from build123d import *

# Parameters (mm, degrees)
F1_DEPTH = 0.635


with BuildPart() as f1:
    # F0 (on Top) → F1 (new body)
    with BuildSketch(Plane.XY):
        with BuildLine():
            Line((-29.810913, 1.540789), (-31.016748, 0))
            Line((-31.016748, 0), (19.896272, 0))
            Line((19.896272, 0), (18.82442, 2.880605))
            Line((18.82442, 2.880605), (17.860188, 5.716184))
            Line((17.860188, 5.716184), (14.670988, 8.373851))
            Line((14.670988, 8.373851), (13.588352, 10.739779))
            ThreePointArc((13.588352, 10.739779), (14.154572, 11.638903), (13.104023, 11.798203))
            Line((13.104023, 11.798203), (12.573407, 12.957779))
            Line((12.573407, 12.957779), (9.713667, 15.340896))
            Line((9.713667, 15.340896), (6.230144, 13.197191))
            Line((6.230144, 13.197191), (3.148568, 11.455429))
            Line((3.148568, 11.455429), (1.540788, 12.795246))
            Line((1.540788, 12.795246), (0.818556, 12.795246))
            ThreePointArc((0.818556, 12.795246), (-4.276831, 15.082857), (-8.518913, 11.449555))
            Line((-8.518913, 11.449555), (-8.641816, 11.589411))
            Line((-8.641816, 11.589411), (-11.991355, 16.680711))
            Line((-11.991355, 16.680711), (-14.938951, 18.288492))
            Line((-14.938951, 18.288492), (-20.432198, 14.269044))
            Line((-20.432198, 14.269044), (-21.582795, 11.795261))
            ThreePointArc((-21.582795, 11.795261), (-22.634312, 11.642479), (-22.073679, 10.739861))
            Line((-22.073679, 10.739861), (-23.11183, 8.507834))
            Line((-23.11183, 8.507834), (-26.059426, 6.364127))
            Line((-26.059426, 6.364127), (-27.265261, 3.148568))
            Line((-27.265261, 3.148568), (-29.810913, 1.540789))
        make_face()
        Polygon((-25.742841, 6.123265), (-22.807967, 8.25772), (-20.128087, 14.019463), (-14.909113, 17.838224), (-12.257344, 16.391804), (-8.96011, 11.380007), (-8.92801, 11.337907), (-5.075081, 6.95354), (-3.355364, 3.514106), (-3.309465, 3.443231), (-0.804003, 0.381), (-30.234767, 0.381), (-29.551596, 1.253941), (-26.9535, 2.894843), align=None, mode=Mode.SUBTRACT)
        with BuildLine():
            Line((-3.717773, 5.090865), (-4.756348, 7.168017))
            Line((-4.756348, 7.168017), (-6.445825, 9.090525))
            Line((-6.445825, 9.090525), (-3.479574, 11.133942))
            Line((-3.479574, 11.133942), (-1.303058, 12.414246))
            Line((-1.303058, 12.414246), (1.402847, 12.414246))
            Line((1.402847, 12.414246), (2.869082, 11.192383))
            Line((2.869082, 11.192383), (-0.923488, 8.639836))
            Line((-0.923488, 8.639836), (-3.616762, 5.088058))
            ThreePointArc((-3.616762, 5.088058), (-3.667275, 5.089198), (-3.717773, 5.090865))
        make_face(mode=Mode.SUBTRACT)
        Polygon((-0.311727, 0.381), (-3.014587, 3.684495), (-3.506604, 4.668528), (-3.313175, 4.85785), (-0.658187, 8.359138), (3.081815, 10.876305), (3.130206, 10.914939), (3.336041, 11.123745), (6.423789, 12.868994), (9.680128, 14.872894), (12.262983, 12.720515), (14.324537, 8.215317), (14.427077, 8.081159), (17.533967, 5.492083), (18.463705, 2.757945), (18.467338, 2.747738), (19.347984, 0.381), align=None, mode=Mode.SUBTRACT)
        with BuildLine():
            ThreePointArc((-21.770268, 11.392193), (-21.766019, 11.363603), (-21.764598, 11.334734))
            ThreePointArc((-21.764598, 11.334734), (-22.351069, 11.305865), (-21.770268, 11.392193))
        make_face(mode=Mode.SUBTRACT)
        with BuildLine():
            Line((-3.684495, 11.455429), (-6.699082, 9.378714))
            Line((-6.699082, 9.378714), (-8.218903, 11.108165))
            ThreePointArc((-8.218903, 11.108165), (-4.466352, 14.664212), (0.353822, 12.795246))
            Line((0.353822, 12.795246), (-1.406807, 12.795246))
            Line((-1.406807, 12.795246), (-3.684495, 11.455429))
        make_face(mode=Mode.SUBTRACT)
        with BuildLine():
            ThreePointArc((13.831154, 11.37468), (13.631239, 11.126505), (13.346187, 11.268991))
            ThreePointArc((13.346187, 11.268991), (13.523069, 11.622855), (13.831154, 11.37468))
        make_face(mode=Mode.SUBTRACT)
    extrude(amount=F1_DEPTH)


solid = f1.part
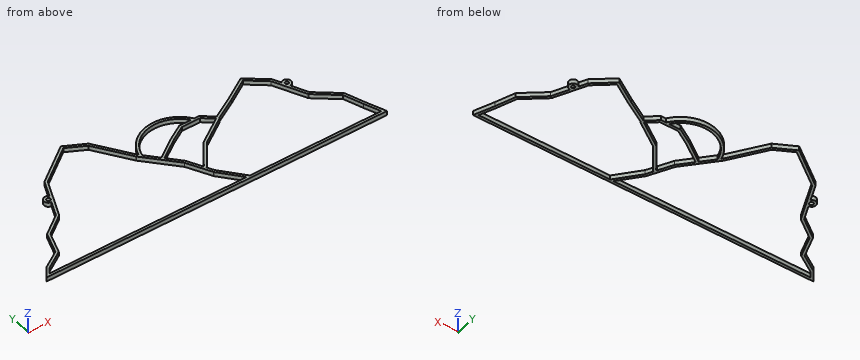
Here's how the part is built. I have some questions about the finished solid (model axes, mm). Coordinates: 2 decimals unless noted, no trailing zeros. Write each loop counter-clockwise with the first axis right and the second up, starting at its lowest first coordinate (ties: lowest second). Pieces come first, ordered by that corner, then holes.
1) If I drill on line 1 (X direction, y = 9.75, z = 0.4); line 2 (Y direction, x = 1, z = 0.45); line 3 (X direction, y = 15.25, z = 0.05), over which ranges is the centre line in solid material (lowest first)?
Filled in:
line 1: x = -22.53 to -22.11, -7.53 to -7.03, -6.16 to -5.49, 0.73 to 1.41, 13.62 to 14.04
line 2: y = 0 to 0.38, 9.48 to 9.93, 12.41 to 12.8
line 3: x = -19.09 to -18.45, -11.51 to -11.05, 9.57 to 9.82
2) If we section it at B-B (z = 0.3): Count the separate pieces of the cut face and the enclosed holes in it, plus the area to 3 significant figures.
Filled in:
separate pieces: 1
enclosed holes: 6
area: 60.8 mm2
3) If we section it at A-A (x = -24.5): List the corners of the cut face in (y, z) for me (3 decimals), plus the area to 3 significant figures.
Filled in:
outline: (0, 0) - (0.381, 0) - (0.381, 0.635) - (0, 0.635) - close; (7.027, 0) - (7.498, 0) - (7.498, 0.635) - (7.027, 0.635) - close
area: 0.541 mm2
4) I'm going to push a flat-ended pin straight in: pin 1 (3 mm diameter, centred on x = -20.5, y = 8, fed in from +Z). Where does the tip first touch, or does it pass through?
Filled in:
pin 1: passes through
